For this review, use the dimensioned drawing (mm, ordinates from the lowest corner) and the shaded views. Round coordinates to 2 decimals unless told otherwise and drop trailing zeros. Order: outer loops, then holes, each group sorted by start corner. A loop starts at its lowest first (then second) coordinate and runs counter-clockwise, first axis right, second up. Notation, with made-up numbers: (30.25, 24.25) -> (39.25, 24.25) arc R28 cw to (39.25, 61.25) -> close; hole circle Ø5 at (-2, 5.25). An arc over 180 degrees is marked (long way). Use a Markdown table: item, result. Add a question column.
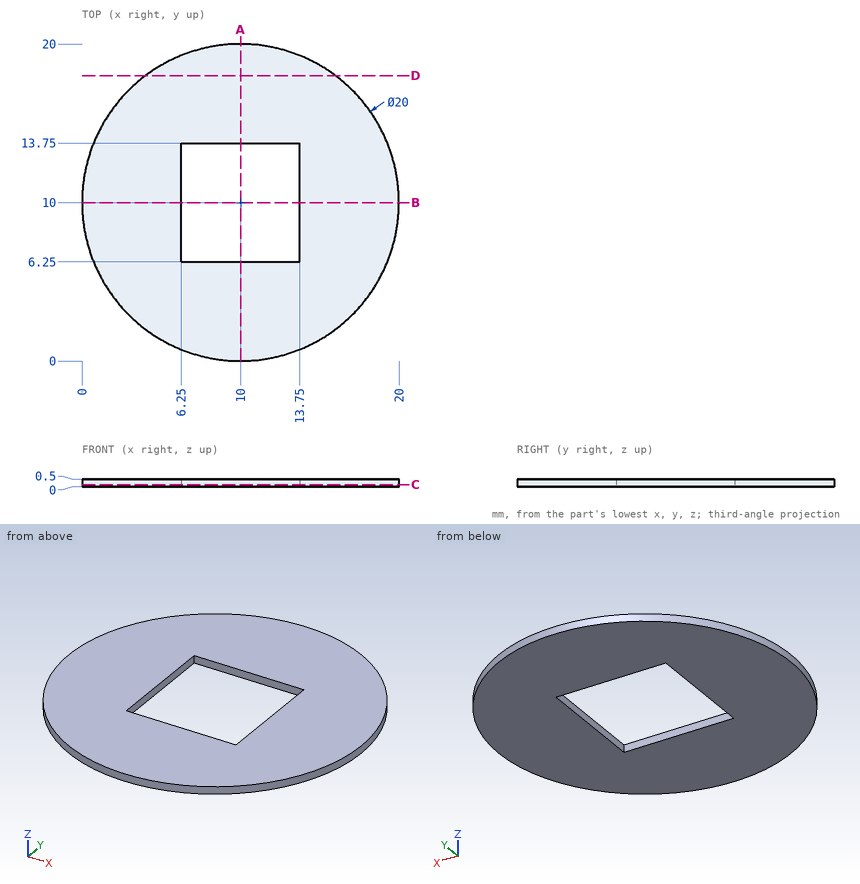
Q1. Insertion check: pin 1 (1 mm diameter, centred on x = 8, y = 3, fed in from -Z). The pin has a flat end and moves straight along its axis. Give the tip position at first contact, or say it passes through.
Q2. Add section C-C (z = 0.15). Write out the cut boundary in (x, y), then the cut area to 3 significant figures.
Q3. Wall thickness on line 1 (X direction, y = 13.25, z = 0.15); line 2 (X direction, y = 12.75, z = 0.4): over which ranges is each line inside the solid? List them lowest first. Write a range as [from, to].
Q4. Add section A-A (x = 10). Write out the cut boundary in (y, z).
Q5. Add section D-D (y = 18). Write out the cut boundary in (x, z).
Report:
| question | item | result |
|---|---|---|
| 1 | pin 1 | stops at z = 0 |
| 2 | outline | circle Ø20 at (10, 10); hole (6.25, 6.25) -> (13.75, 6.25) -> (13.75, 13.75) -> (6.25, 13.75) -> close |
| 2 | area | 258 mm² |
| 3 | line 1 | x = [0.54, 6.25], [13.75, 19.46] |
| 3 | line 2 | x = [0.39, 6.25], [13.75, 19.61] |
| 4 | outline | (0, 0) -> (6.25, 0) -> (6.25, 0.5) -> (0, 0.5) -> close; (13.75, 0) -> (20, 0) -> (20, 0.5) -> (13.75, 0.5) -> close |
| 5 | outline | (4, 0) -> (16, 0) -> (16, 0.5) -> (4, 0.5) -> close |
